Work out the finished part from the listing and answer in its coordinate system (mm). Face numbers are marked on the shaded views. A direction names the side the tool comes from. Round coordinates to 2 decimals unless told otherwise and drop trailing zeros. Write each loop counter-clockwise with the first axis right and the second up, starting at its lowest first coordinate (ties: lowest second). Pieces come first, ordered by that corner, then holes.
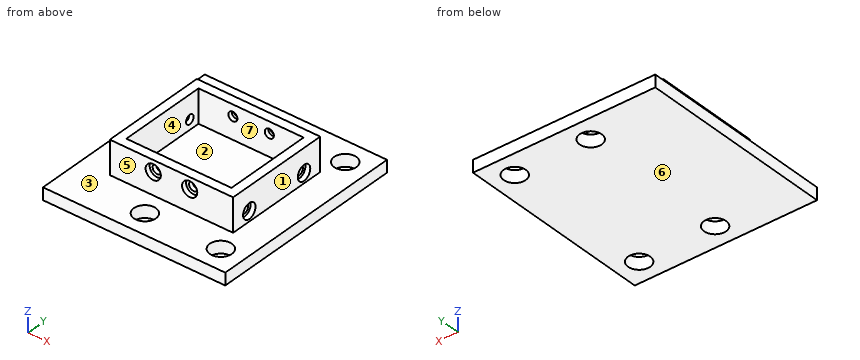
from build123d import *

# Parameters (mm, degrees)
SKETCH_1_W          = 60
SKETCH_1_H          = 65
SKETCH_1_R          = 3.625
EXTRUDE_1_DEPTH     = 4
SKETCH_2_W          = 40.6
SKETCH_2_H          = 35
SKETCH_2_W_2        = 34.6
SKETCH_2_H_2        = 29
EXTRUDE_2_DEPTH     = 11
SKETCH_3_R          = 1.5
CUT_EXTRUDE_1_DEPTH = 51
SKETCH_4_R          = 2.5
CUT_EXTRUDE_2_DEPTH = 1.6
SKETCH_5_R          = 1.5
CUT_EXTRUDE_3_DEPTH = 51.3
SKETCH_6_R          = 2.5
CUT_EXTRUDE_4_DEPTH = 1.6


with BuildPart() as part:
    # 스케치1 → 보스-돌출1 (new body)
    with BuildSketch(Plane.XY):
        Rectangle(SKETCH_1_W, SKETCH_1_H)
        with Locations((-2.6, 25)):
            Circle(SKETCH_1_R, mode=Mode.SUBTRACT)
        with Locations((-2.6, -25)):
            Circle(SKETCH_1_R, mode=Mode.SUBTRACT)
        with Locations((22.4, 25)):
            Circle(SKETCH_1_R, mode=Mode.SUBTRACT)
        with Locations((22.4, -25)):
            Circle(SKETCH_1_R, mode=Mode.SUBTRACT)
    extrude(amount=EXTRUDE_1_DEPTH)

    # 스케치2 → 보스-돌출2 (add)
    with BuildSketch(Plane.XY.offset(4)):
        Rectangle(SKETCH_2_W, SKETCH_2_H)
        Rectangle(SKETCH_2_W_2, SKETCH_2_H_2, mode=Mode.SUBTRACT)
    extrude(amount=EXTRUDE_2_DEPTH)

    # 스케치3 → 컷-돌출1 (cut, through all)
    with BuildSketch(Plane.XZ.offset(17.5)):
        with Locations((-6, 11.25)):
            Circle(SKETCH_3_R)
        with Locations((6, 11.25)):
            Circle(SKETCH_3_R)
    extrude(amount=-CUT_EXTRUDE_1_DEPTH, mode=Mode.SUBTRACT)

    # 스케치4 → 컷-돌출2 (cut)
    with BuildSketch(Plane.XZ.offset(17.5)):
        with Locations((-6, 11.25)):
            Circle(SKETCH_4_R)
        with Locations((6, 11.25)):
            Circle(SKETCH_4_R)
    cut_extrude_2 = extrude(amount=-CUT_EXTRUDE_2_DEPTH, mode=Mode.SUBTRACT)

    # 대칭 복사1: 컷-돌출2 across plane
    add(cut_extrude_2.mirror(Plane.ZX), mode=Mode.SUBTRACT)

    # 스케치5 → 컷-돌출3 (cut, through all)
    with BuildSketch(Plane.ZY.offset(20.3)):
        with Locations((7.25, -11)):
            Circle(SKETCH_5_R)
        with Locations((7.25, 11)):
            Circle(SKETCH_5_R)
    extrude(amount=-CUT_EXTRUDE_3_DEPTH, mode=Mode.SUBTRACT)

    # 스케치6 → 컷-돌출4 (cut)
    with BuildSketch(Plane.ZY.offset(20.3)):
        with Locations((7.25, 11)):
            Circle(SKETCH_6_R)
        with Locations((7.25, -11)):
            Circle(SKETCH_6_R)
    cut_extrude_4 = extrude(amount=-CUT_EXTRUDE_4_DEPTH, mode=Mode.SUBTRACT)

    # 대칭 복사2: 컷-돌출4 across plane
    add(cut_extrude_4.mirror(Plane(origin=(0, 0, 0), x_dir=(0, 0, 1), z_dir=(1, 0, 0))), mode=Mode.SUBTRACT)


solid = part.part
Q1. Find section D-D (y = -3.5). Determine the outline of the cut face in (x, z).
Q2. Given pin 1 (2 mm diameter, centred on y = -5, z = 4.5, fed in from -X); pin 2 (4 mm diameter, centred on y = -10.5, z = 7, fed in from +X); pin 3 (8 mm diameter, centred on x = -6, z = 11.25, fed in from -Y); pin 4 (1.5 mm diameter, centred on x = 17, z = 6.5, fed in from +Y), each flat-ended and moving along its own axis, determine where each tip first touches the part or whether it passes through.
Q3. Find section C-C (z = 1). Determine the outline of the cut face in (x, y) (3 decimals), plus the area to 3 significant figures.
Q4. Find the intervals of material crossed by L1, parallel to Y at x = -19.7, z = 7.25; L2, parallel to X at y = 4, z = 7.75; L3, parallel to Z at x = -6, y = -15, in increasing order.
Q5. The mould has two halves that part along X. Classify the marked faces 1, 2, 3 and 4: +X half, -X half, draft (parallel to the pull), parting line (faces both ways), or undercut.
Q6. Find section B-B (y = -25). Determine the outline of the cut face in (x, z) (3 decimals), plus the area to 3 significant figures.
Q7. Find section A-A (x = -2.6). Determine the outline of the cut face in (y, z) (3 decimals).
Q8. A tool of negligible diameter and unlimited length cuts with its end or side. For the marked faces 5, 6 and 7, from which of +Z, -Z, +X, -X, +Y, -Y can it reach the whole face along a straight path? Write none if from no direction.
Report:
1. outline: (-30, 0) - (30, 0) - (30, 4) - (20.3, 4) - (20.3, 15) - (17.3, 15) - (17.3, 4) - (-17.3, 4) - (-17.3, 15) - (-20.3, 15) - (-20.3, 4) - (-30, 4) - close
2. pin 1: stops at x = -30
2. pin 2: stops at x = 20.3
2. pin 3: stops at y = -17.5
2. pin 4: stops at y = 17.5
3. outline: (-30, -32.5) - (30, -32.5) - (30, 32.5) - (-30, 32.5) - close; hole circle Ø7.25 at (-2.6, -25); hole circle Ø7.25 at (-2.6, 25); hole circle Ø7.25 at (22.4, -25); hole circle Ø7.25 at (22.4, 25)
3. area: 3,730 mm2
4. L1: y = -17.5 to -13.5, -8.5 to 8.5, 13.5 to 17.5
4. L2: x = -20.3 to -17.3, 17.3 to 20.3
4. L3: z = 0 to 9.75, 12.75 to 15
5. face 1: +X half
5. face 2: undercut
5. face 3: draft
5. face 4: undercut
6. outline: (-30, 0) - (-6.225, 0) - (-6.225, 4) - (-30, 4) - close; (1.025, 0) - (18.775, 0) - (18.775, 4) - (1.025, 4) - close; (26.025, 0) - (30, 0) - (30, 4) - (26.025, 4) - close
6. area: 182 mm2
7. outline: (-32.5, 0) - (-28.625, 0) - (-28.625, 4) - (-32.5, 4) - close; (-21.375, 0) - (21.375, 0) - (21.375, 4) - (17.5, 4) - (17.5, 15) - (14.5, 15) - (14.5, 4) - (-14.5, 4) - (-14.5, 15) - (-17.5, 15) - (-17.5, 4) - (-21.375, 4) - close; (28.625, 0) - (32.5, 0) - (32.5, 4) - (28.625, 4) - close
8. face 5: +Z, +X, -X, -Y
8. face 6: -Z, +X, -X, +Y, -Y
8. face 7: +Z
